Answer from the drawing. Dimensions are ordinates in mm from the lowest x, y and z of the part. Coordinates: 2 decimals unless noted, no trailing zeros. Order: outer loops, then holes, each group sorted by start corner. A loop starts at its lowest first (then second) coordinate and runs counter-clockwise, first axis right, second up. Notation, with made-up numbers: M 13.5,8.25 L 48.5,8.25 A21 ccw 48.5,15.25 Z; hole C 65,43 d5. An arc over 180 degrees is marked long. One line per question, with ' | ' between items. Start each with the question number.
1) Find section D-D, the plane x = 45. Write down the section's boundary in (y, z).
2) Consider probe 1 along Y at (x, z) = (139.7, 8.75) (3 decimals); probe 2 along X at (y, z) = (88.5, 22). Determine where each line is inside the solid, lowest interval first.
3) Find section C-C, the plane x = 107.95. Write down the section's boundary in (y, z) (3 decimals).
4) Given P1, Ø5.5, axis at x = 12.7, y = 12.7, coming from the +Z side, flat-ended and moving along its own axis, determine where the tip first touches the part or whether it passes through.
5) Find section A-A, the plane z = 12.25. Count the separate pieces of the cut face and the enclosed holes in it, plus the area to 3 significant figures.
6) Find section B-B, the plane y = 50.8. Write down the section's boundary in (x, z) (3 decimals), plus the area to 3 significant figures.
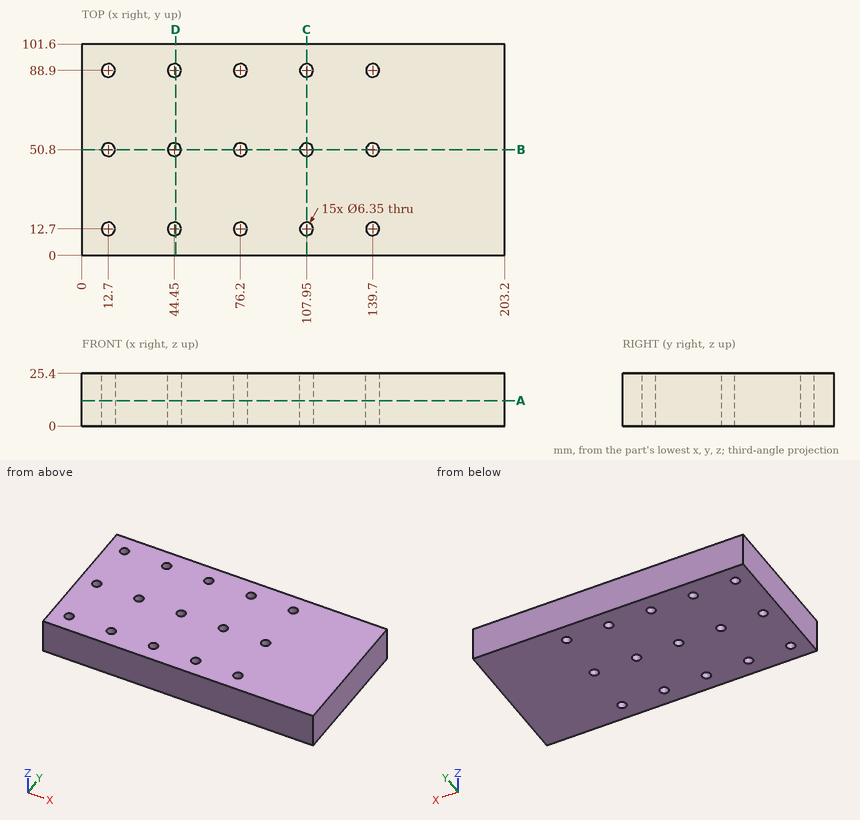
Report:
1) outline: M 0,0 L 9.57,0 L 9.57,25.4 L 0,25.4 Z; M 15.83,0 L 47.67,0 L 47.67,25.4 L 15.83,25.4 Z; M 53.93,0 L 85.77,0 L 85.77,25.4 L 53.93,25.4 Z; M 92.03,0 L 101.6,0 L 101.6,25.4 L 92.03,25.4 Z
2) probe 1: y = 0 to 9.525, 15.875 to 47.625, 53.975 to 85.725, 92.075 to 101.6 | probe 2: x = 0 to 9.55, 15.85 to 41.3, 47.6 to 73.05, 79.35 to 104.8, 111.1 to 136.55, 142.85 to 203.2
3) outline: M 0,0 L 9.525,0 L 9.525,25.4 L 0,25.4 Z; M 15.875,0 L 47.625,0 L 47.625,25.4 L 15.875,25.4 Z; M 53.975,0 L 85.725,0 L 85.725,25.4 L 53.975,25.4 Z; M 92.075,0 L 101.6,0 L 101.6,25.4 L 92.075,25.4 Z
4) P1: passes through
5) separate pieces: 1 | enclosed holes: 15 | area: 20,200 mm^2
6) outline: M 0,0 L 9.525,0 L 9.525,25.4 L 0,25.4 Z; M 15.875,0 L 41.275,0 L 41.275,25.4 L 15.875,25.4 Z; M 47.625,0 L 73.025,0 L 73.025,25.4 L 47.625,25.4 Z; M 79.375,0 L 104.775,0 L 104.775,25.4 L 79.375,25.4 Z; M 111.125,0 L 136.525,0 L 136.525,25.4 L 111.125,25.4 Z; M 142.875,0 L 203.2,0 L 203.2,25.4 L 142.875,25.4 Z | area: 4,350 mm^2
